```python
from build123d import *

# Parameters (mm, degrees)
SKETCH1_W           = 160
SKETCH1_H           = 90
BOSS_EXTRUDE1_DEPTH = 2.5
SKETCH2_W           = 160
SKETCH2_H           = 90
SKETCH2_W_2         = 156
SKETCH2_H_2         = 86
BOSS_EXTRUDE2_DEPTH = 1.5
SKETCH3_R           = 27.5
BOSS_EXTRUDE3_DEPTH = 2.5


with BuildPart() as part:
    # Sketch1 → Boss-Extrude1 (new body, symmetric)
    with BuildSketch(Plane.XY):
        Rectangle(SKETCH1_W, SKETCH1_H)
    extrude(amount=BOSS_EXTRUDE1_DEPTH, both=True)

    # Sketch2 → Boss-Extrude2 (add)
    with BuildSketch(Plane.XY.offset(2.5)):
        Rectangle(SKETCH2_W, SKETCH2_H)
        Rectangle(SKETCH2_W_2, SKETCH2_H_2, mode=Mode.SUBTRACT)
    extrude(amount=BOSS_EXTRUDE2_DEPTH)



with BuildPart() as body_2:
    # Sketch3 → Boss-Extrude3 (new body)
    with BuildSketch(Plane(origin=(0, -60, 0), x_dir=(1, 0, 0), z_dir=(0, 1, 0))):
        with Locations((0, 5)):
            Circle(SKETCH3_R)
    extrude(amount=BOSS_EXTRUDE3_DEPTH)


with BuildPart() as part_1:
    add(part.part)

    add(body_2.part)  # Loft1 merges body 2
    # Sketch5 → Loft1 section 0
    with BuildSketch(Plane(origin=(0, 0, -2.5), x_dir=(-1, 0, 0), z_dir=(0, 0, -1))):
        Polygon((0, -22.5), (-5, -37.5), (5, -37.5), align=None)
    # Sketch4 → Loft1 section 1
    with BuildSketch(Plane(origin=(0, -57.5, 0), x_dir=(1, 0, 0), z_dir=(0, 1, 0))):
        Polygon((-5, 7.5), (0, 19.5), (5, 7.5), align=None)
    loft()


solid = part_1.part
```
Source: CAD feature listing. Evaluate the final solid. Frame: model axes, mm. A direction names the side the tool comes from. Round coordinates to 2 decimals unless told otherwise and drop trailing zeros. Loops run counter-clockwise (first coordinate to the right, second up) from the corner with the lowest first, then second, coordinate; pieces in that order, holes last. Notation, with made-up numbers: M 26.25,1.25 L 37.25,1.25 A10 cw 37.25,11.25 Z; hole C 35.25,2.25 d5. An arc over 180 degrees is marked long. Use a Markdown table: item, result. Add a question column.
1. Line query: line 1 (Z direction, x = -10, y = 20.5); line 2 (Y direction, x = 15.5, z = -11); line 3 (Z direction, x = 23.5, y = -44). Output: solid intervals per line, ascending.
2. Mould query, pull axis Z, two halves, no side actions, for faces 1 (the flat face through (0.07, -47.64, -5.035)), 2 (the flat face through (-1, 45, 1)), 3 (the flat face through (0, 44, 4)), 4 (the cylindrical face through (-21.823, -58.768, 11.733)). Classes: pulls with the +Z half, pulls with the -Z half, needs draft (parallel to the pull), parting line crosses it, or undercut.
3. Contact query for flat-ended pins moving along their axis: P1, Ø8, axis at x = -24, z = -11, coming from the +Y side; P2, Ø2, axis at x = 55.5, y = 23, coming from the -Z side; P3, Ø8, axis at y = 14.5, z = 7.5, coming from the -X side. Output: stop coordinate, or through.
4. Section query C-C on y = -20. Return the cut outline in (x, z).
5. Section query A-A on x = -8. Return the cut outline in (y, z).
6. Section query D-D on z = 11.5. Return the cut outline in (x, y), then the cut area to 3 significant figures.
7. Section query B-B on x = 48. Return the cut outline in (y, z).
8. Reachability of faces 5 (the flat face through (-1, 1, 2.5)), 6 (the flat face through (-80, -1, 1)) from +Z, -Z, +X, -X, +Y, -Y: full face, straight path, thin tool, end or side. Return the list, or none.
Reported:
| question | item | result |
|---|---|---|
| 1 | line 1 | z = -2.5 to 2.5 |
| 1 | line 2 | y = -60 to -57.5 |
| 1 | line 3 | z = -2.5 to 4 |
| 2 | face 1 | undercut |
| 2 | face 2 | needs draft |
| 2 | face 3 | pulls with the +Z half |
| 2 | face 4 | parting line crosses it |
| 3 | P1 | stops at y = -57.5 |
| 3 | P2 | stops at z = -2.5 |
| 3 | P3 | stops at x = -80 |
| 4 | outline | M -80,-2.5 L 80,-2.5 L 80,4 L 78,4 L 78,2.5 L -78,2.5 L -78,4 L -80,4 Z |
| 5 | outline | M -60,-31.31 L -57.5,-31.31 L -57.5,21.31 L -60,21.31 Z; M -45,-2.5 L 45,-2.5 L 45,4 L 43,4 L 43,2.5 L -43,2.5 L -43,4 L -45,4 Z |
| 6 | outline | M -22,-60 L 22,-60 L 22,-57.5 L -22,-57.5 Z |
| 6 | area | 110 mm² |
| 7 | outline | M -45,-2.5 L 45,-2.5 L 45,4 L 43,4 L 43,2.5 L -43,2.5 L -43,4 L -45,4 Z |
| 8 | face 5 | +Z |
| 8 | face 6 | +Z, -Z, -X, +Y, -Y |
